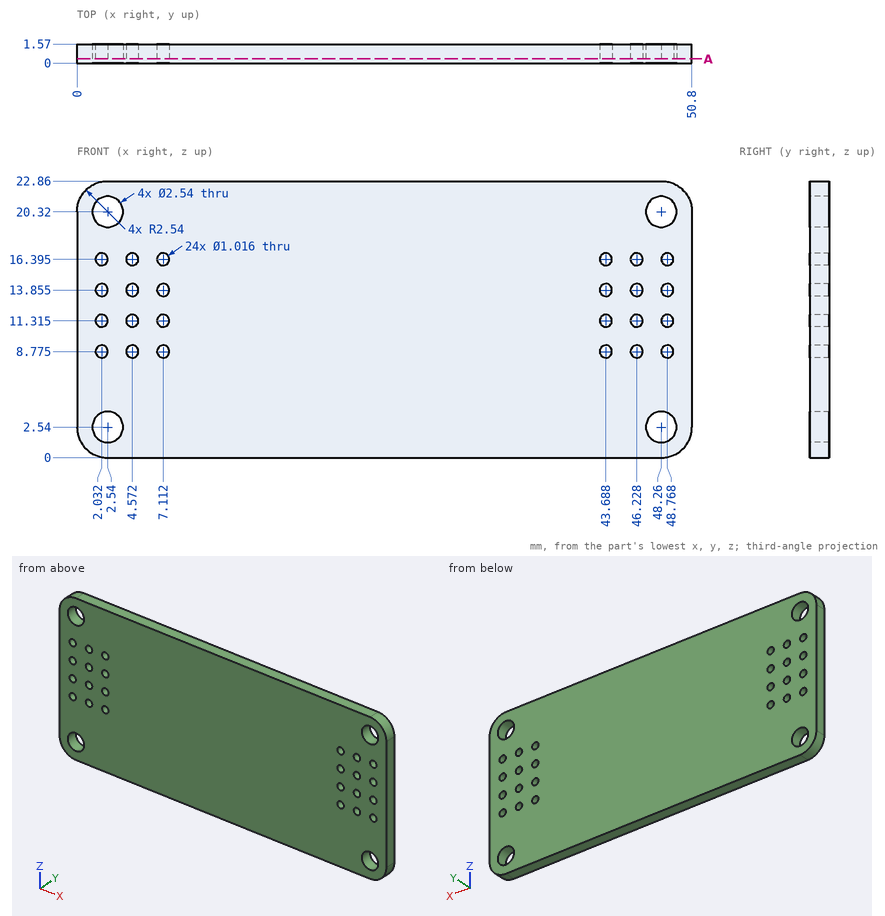
Study the drawing (mm; zero at the part's minimum x, y, z) and answer. Coordinates: 2 decimals unless noted, no trailing zeros. Answer in a Markdown table with one row per item. Add a question column.
Item 1: This flat-tipped pin is pushed along its axis until it touches: P1, Ø0.6, axis at x = 4.57, z = 16.4, coming from the +Y side. Where does it stop, or does it pass through?
Item 2: Find the intervals of material crossed by L1, parallel to X at y = 0.65, z = 20.25; L2, parallel to X at y = 0.75, z = 21; L3, parallel to Z at x = 3, y = 0.5 (1 decimal), in increasing order. Write a range as from..to.
Item 3: Find section A-A (y = 0.35). State how many separate pieces and enclosed holes the cut face has, then the cut area to 3 significant figures.
Result set:
| question | item | result |
|---|---|---|
| 1 | P1 | passes through |
| 2 | L1 | x = 0..1.27, 3.81..46.99, 49.53..50.8 |
| 2 | L2 | x = 0.09..1.47, 3.61..47.19, 49.33..50.71 |
| 2 | L3 | z = 0..1.4, 3.7..19.1, 21.5..22.9 |
| 3 | separate pieces | 1 |
| 3 | enclosed holes | 28 |
| 3 | area | 1,120 mm² |
